from build123d import *

# Parameters (mm, degrees)
BOSS_EXTRUDE1_DEPTH = 2.4
SKETCH8_R           = 1.5
CUT_EXTRUDE1_DEPTH  = 5.837957558


with BuildPart() as part:
    # Sketch1 → Boss-Extrude1 (new body)
    with BuildSketch(Plane(origin=(0, 0, 0), x_dir=(0, 0, -1), z_dir=(1, 0, 0))):
        Polygon((0, 3.175426481), (-2.75, 1.58771324), (-2.75, -1.58771324), (0, -3.175426481), (2.75, -1.58771324), (2.75, 1.58771324), align=None)
    extrude(amount=-BOSS_EXTRUDE1_DEPTH)

    # Sketch2 → Cut-Revolve1 (revolve, cut)
    with BuildSketch(Plane.XY):
        Polygon((-2.4, 2.75), (-2.154379907, 3.175426481), (-2.4, 3.175426481), align=None)
    revolve(axis=Axis((-2.23854625, 0, 0), (1, 0, 0)), mode=Mode.SUBTRACT)

    # Sketch8 → Cut-Extrude1 (cut, through all)
    with BuildSketch(Plane(origin=(0, 0, 0), x_dir=(0, 0, -1), z_dir=(1, 0, 0))):
        Circle(SKETCH8_R)
    extrude(amount=-CUT_EXTRUDE1_DEPTH, mode=Mode.SUBTRACT)


solid = part.part
Build history of the part. All positions in model axes, mm. Give positions to 0.01 mm unless a question says otherwise; leave off trailing zeros. Order: outer loops, then holes, each group sorted by start corner. A loop starts at its lowest first (then second) coordinate and runs counter-clockwise, first axis right, second up. Notation, with made-up numbers: M -13,-22.75 L 22,-22.75 A14 cw 22,1.25 Z; hole C 28,42.25 d9. An arc over 180 degrees is marked long. Use one line per item in the form item = value.
1) Probe probe 1 along Y at (x, z) = (-1.55, -1); probe 2 along Z at (x, y) = (-0.45, 1); probe 3 along Z at (x, y) = (-1.7, -0.75). List the from-to ranges inside material, lowest first.
Calculated:
probe_1 = -2.6 to -1.12, 1.12 to 2.6
probe_2 = -2.75 to -1.12, 1.12 to 2.75
probe_3 = -2.75 to -1.3, 1.3 to 2.75
2) Two-plate mould, pull along Y, no slides. Class faces 1 (the face through (-2.4, -1.2, -1.2)), 2 (the face through (-1.18, 0.07, 1.5)), 3 (the face through (-2.31, -1.46, -2.51)): released by +Y, released by -Y, zero draft, split by the parting line, or undercut.
Calculated:
face_1 = zero draft
face_2 = undercut
face_3 = released by -Y
3) Saw through at A-A (x = -0.25). Give the cut face in (y, z), plus the area to 3 significant figures.
Calculated:
outline = M -3.18,0 L -1.59,-2.75 L 1.59,-2.75 L 3.18,0 L 1.59,2.75 L -1.59,2.75 Z; hole C 0,0 d3
area = 19.1 mm2
